Check sheet for the modelled part. Datum: model origin and axes. Units: mm. A direction names the side the tool comes from. Round coordinates to 2 decimals unless told otherwise and drop trailing zeros. Order: outer loops, then holes, each group sorted by start corner. A loop starts at its lowest first (then second) coordinate and runs counter-clockwise, first axis right, second up. Notation, with made-up numbers: (47.25, 22.25) -> (98.25, 22.25) arc R21 cw to (98.25, 38.25) -> close; hole circle Ø11 at (84.25, 73.5). An arc over 180 degrees is marked (long way). Answer in a Markdown table with one row per item. Add a question column.
1. Depth check by flat-ended pin: P1, Ø12, axis at x = -69, z = -38, coming from the -Y side; P2, Ø1.5, axis at x = -54, y = 2, coming from the +Z side (3 decimals); P3, Ø2, axis at y = 1.5, z = -46, coming from the +X side; P4, Ø2, axis at y = 5, z = -44.5, coming from the +X side. Enter the tip coordinate at first touch or a pass-through.
2. Sectioned sample at D-D, the plane y = 2.25. Record the boundary of the cut face in (x, z).
3. Access from +Z, -Z, +X, -X, +Y, -Y to the whole of each face (thin tool, end or side, straight path). Record for faces 4 (the flat face through (-69.65, 5.03, -20.85)), 5 (the flat face through (-70, 1, -27)), 6 (the flat face through (-27.592, 5.028, -52.725)).
4. Draft check along Z on faces 1 (the flat face through (-32.5, 3, -56.4)), 2 (the flat face through (-29, 7, -21)), 3 (the flat face through (-35.91, 5.03, -60.4)). Enter one of: +Z half, -Z half, draft (parallel to the pull), parting line (faces both ways), or undercut.
5. Sectioned sample at C-C, the plane z = -20.5. Record the boundary of the cut face in (x, y).
6. Material ranges on L1, parallel to Z at x = -50, y = 5; L2, parallel to X at y = 0.75, z = -38; L3, parallel to Z at x = -43.5, y = 5.5, recorded low to high. Write a range as from..to.
7. Sectioned sample at B-B, the plane x = -70. Record the boundary of the cut face in (y, z), then the cut area to 3 significant figures.
8. Sectioned sample at A-A, the plane y = 5.75. Record the boundary of the cut face in (x, z).
```python
from build123d import *

# Parameters (mm, degrees)
ESQUISSE6_R             = 28
BOSS_EXTRU_3_DEPTH      = 3
ESQUISSE7_R             = 27
ESQUISSE7_R_2           = 26
BOSS_EXTRU_4_DEPTH      = 4
ESQUISSE8_R             = 25
ENL_V_MAT_EXTRU_2_DEPTH = 2
ESQUISSE9_R             = 23
ENL_V_MAT_EXTRU_3_DEPTH = 102.549659352
ENL_V_MAT_EXTRU_4_DEPTH = 4


with BuildPart() as part:
    # Esquisse6 → Boss.-Extru.3 (new body)
    with BuildSketch(Plane(origin=(0, 0, 0), x_dir=(1, 0, 0), z_dir=(0, 1, 0))):
        with Locations(Location((-49.260149918, 37.629281188, 0), (0, 0, 270))):
            Circle(ESQUISSE6_R)
    extrude(amount=BOSS_EXTRU_3_DEPTH)

    # Esquisse7 → Boss.-Extru.4 (add)
    with BuildSketch(Plane(origin=(0, 3, 0), x_dir=(1, 0, 0), z_dir=(0, 1, 0))):
        with Locations(Location((-49.260149918, 37.629281188, 0), (0, 0, 270))):
            Circle(ESQUISSE7_R)
        with Locations(Location((-49.260149918, 37.629281188, 0), (0, 0, 270))):
            Circle(ESQUISSE7_R_2, mode=Mode.SUBTRACT)
    extrude(amount=BOSS_EXTRU_4_DEPTH)

    # Esquisse8 → Enlèv. mat.-Extru.2 (cut)
    with BuildSketch(Plane(origin=(0, 3, 0), x_dir=(1, 0, 0), z_dir=(0, 1, 0))):
        with Locations(Location((-49.260149918, 37.629281188, 0), (0, 0, 270))):
            Circle(ESQUISSE8_R)
    extrude(amount=-ENL_V_MAT_EXTRU_2_DEPTH, mode=Mode.SUBTRACT)

    # Esquisse9 → Enlèv. mat.-Extru.3 (cut, through all)
    with BuildSketch(Plane(origin=(0, 1, 0), x_dir=(1, 0, 0), z_dir=(0, 1, 0))):
        with Locations(Location((-49.260149918, 37.629281188, 0), (0, 0, 270))):
            Circle(ESQUISSE9_R)
    extrude(amount=-ENL_V_MAT_EXTRU_3_DEPTH, mode=Mode.SUBTRACT)

    # Esquisse10 → Enlèv. mat.-Extru.4 (cut)
    with BuildSketch(Plane(origin=(0, 7, 0), x_dir=(1, 0, 0), z_dir=(0, 1, 0))):
        Polygon((-71.468932312, 22.27447788), (-58.878892443, 12.400730055), (-61.579583758, 8.957071992), (-74.169623626, 18.830819817), align=None)
        Polygon((-22.927613797, 54.376268132), (-25.894954155, 51.159529779), (-37.65537385, 62.00814852), (-34.688033492, 65.224886873), align=None)
    extrude(amount=-ENL_V_MAT_EXTRU_4_DEPTH, mode=Mode.SUBTRACT)


solid = part.part
```
Answer key:
| question | item | result |
|---|---|---|
| 1 | P1 | stops at y = 0 |
| 1 | P2 | stops at z = -9.915 |
| 1 | P3 | stops at x = -22.25 |
| 1 | P4 | stops at x = -22.91 |
| 2 | outline | circle Ø56 at (-49.26, -37.63); hole circle Ø50 at (-49.26, -37.63) |
| 3 | face 4 | +Z, -X, +Y |
| 3 | face 5 | +Y |
| 3 | face 6 | -Z, +X, +Y |
| 4 | face 1 | undercut |
| 4 | face 2 | draft |
| 4 | face 3 | -Z half |
| 5 | outline | (-71.41, 0) -> (-64.61, 0) -> (-64.61, 1) -> (-67.47, 1) -> (-67.47, 3) -> (-68.82, 3) -> (-68.82, 7) -> (-69.21, 7) -> (-69.21, 3) -> (-71.41, 3) -> close; (-33.91, 0) -> (-27.11, 0) -> (-27.11, 3) -> (-28.39, 3) -> (-28.39, 7) -> (-29.7, 7) -> (-29.7, 3) -> (-31.05, 3) -> (-31.05, 1) -> (-33.91, 1) -> close |
| 6 | L1 | z = -64.62..-63.62, -11.64..-10.64 |
| 6 | L2 | x = -77.26..-72.26, -26.26..-21.26 |
| 6 | L3 | z = -64.01..-62.98, -12.28..-11.25 |
| 7 | outline | (0, -56.44) -> (3, -56.44) -> (3, -54.92) -> (7, -54.92) -> (7, -53.31) -> (3, -53.31) -> (3, -51.59) -> (1, -51.59) -> (1, -47.57) -> (0, -47.57) -> close; (0, -27.69) -> (1, -27.69) -> (1, -23.67) -> (3, -23.67) -> (3, -21.95) -> (7, -21.95) -> (7, -21.12) -> (3, -21.12) -> (3, -18.82) -> (0, -18.82) -> close |
| 7 | area | 46.9 mm² |
| 8 | outline | (-71.47, -22.27) arc R27 ccw to (-37.66, -62.01) -> (-34.21, -58.83) arc R26 cw to (-67.78, -19.38) -> close; (-62.56, -15.29) arc R26 cw to (-29.34, -54.34) -> (-25.89, -51.16) arc R27 ccw to (-58.88, -12.4) -> close |
